Read the model definition and answer for the solid it produces. Units are mm, in the model's axes. Face numbers are marked on the shaded views. A direction names the side the tool comes from. Coordinates: 2 decimals unless noted, no trailing zeros. Loops run counter-clockwise (first coordinate to the right, second up) from the corner with the lowest first, then second, coordinate; pieces in that order, holes last. Notation, with made-up numbers: (-12.75, 9.25) - (16.25, 9.25) arc R20 ccw to (16.25, 48.25) - close; hole circle Ø3 at (12, 64.5). An arc over 180 degrees is marked (long way). Use one line per item in the form item = value. Start each with the question number.
1) Which of the six approach directions +Z, -Z, +X, -X, +Y, -Y give full straight-line access (tool end or side, diameter ignored) to the marked faces 4 and 5?
2) Each of these flat-tipped pins is pushed along its axis until it touches: P1, Ø2, axis at x = -16.5, z = 5, coming from the -Y side; P2, Ø3, axis at y = -17.5, z = 5, coming from the +X side; P3, Ø6, axis at x = -22.5, y = -20, coming from the -Z side. Where does it stop, or does it pass through?
3) Consider line 1 (Y direction, x = -3, z = 2.25); line 2 (Z direction, x = 24, y = 4); line 3 (Y direction, x = 0, z = 4.25). Determine where each line is inside the solid, lowest interval first.
4) The mould has two halves that part along X. Classify the marked faces 1, 2 and 3: released by +X, released by -X, zero draft, split by the parting line, or undercut.
5) A cutting plane is placed at C-C (z = 3). Give the vertices of the cut face in (x, y), and give its area (3 significant figures).
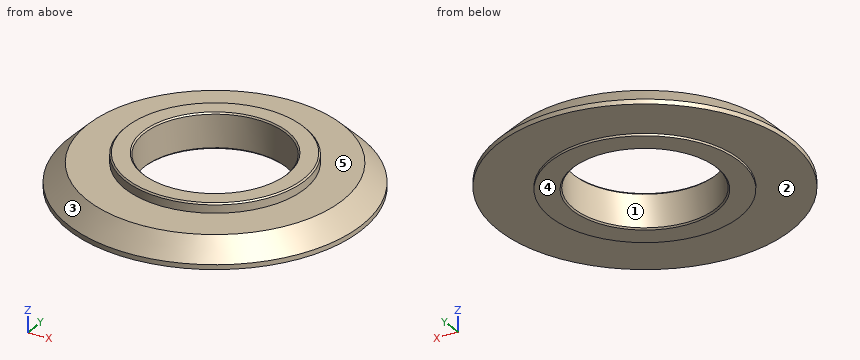
Autodesk Inventor part; units mm, degrees
ref_plane "YZ Plane" through (0, 0, 0) normal (1, 0, 0) x (0, 1, 0)
ref_plane "XZ Plane" through (0, 0, 0) normal (0, 1, 0) x (-1, 0, 0)
ref_plane "XY Plane" through (0, 0, 0) normal (0, 0, 1) x (1, 0, 0)
sketch "草圖1" plane through (0, 0, 0) normal (0, 0, 1) x (1, 0, 0)
  circle A0 centre (0, 0) radius 31
  dimension "d0" = 62
extrude "擠出1" add sketch "草圖1" along normal blind 1
sketch "草圖2" plane through (0, 0, 1) normal (0, 0, 1) x (1, 0, 0)
  circle A0 centre (0, 0) radius 31
  circle A1 centre (0, 0) radius 27
  dimension "d3" = 54
extrude "擠出2" add sketch "草圖2" along normal blind 4 contours A1
sketch "草圖3" plane through (0, 0, 5) normal (0, 0, 1) x (1, 0, 0)
  circle A0 centre (0, 0) radius 27
  circle A1 centre (0, 0) radius 19
  dimension "d6" = 38
extrude "擠出3" add sketch "草圖3" along normal blind 2 contours A1
sketch "草圖4" plane through (0, 0, 0) normal (0, 0, -1) x (-1, 0, 0)
  circle A0 centre (0, 0) radius 31
  circle A1 centre (0, 0) radius 20
  dimension "d9" = 40
extrude "擠出4" add sketch "草圖4" along normal blind 0.5 contours A1
sketch "草圖5" plane through (0, 0, 7) normal (0, 0, 1) x (1, 0, 0)
  circle A0 centre (0, 0) radius 19
  circle A1 centre (0, 0) radius 15
  dimension "d12" = 30
extrude "擠出5" cut sketch "草圖5" against normal through all contours A1
chamfer "倒角1" distance 4 angle 45 1 edges at (-27, 0, 1)
chamfer "倒角2" distance 0.3 angle 45 3 edges at (-15, 0, 7) (-15, 0, -0.5) (-19, 0, 7)
properties part number "KM-20140709-07-Kashiyama 機械油封墊片(T=7.5)"
Found:
q1.face_4 = -Z, +X, -X, +Y, -Y
q1.face_5 = +Z
q2.P1 = -22.81
q2.P2 = 22.81
q2.P3 = 0
q3.line_1 = -29.6 to -14.7, 14.7 to 29.6
q3.line_2 = 0 to 5
q3.line_3 = -27.75 to -15, 15 to 27.75
q4.face_1 = undercut
q4.face_2 = zero draft
q4.face_3 = split by the parting line
q5.outline = circle Ø58 at (0, 0); hole circle Ø30 at (0, 0)
q5.area = 1,940 mm^2
